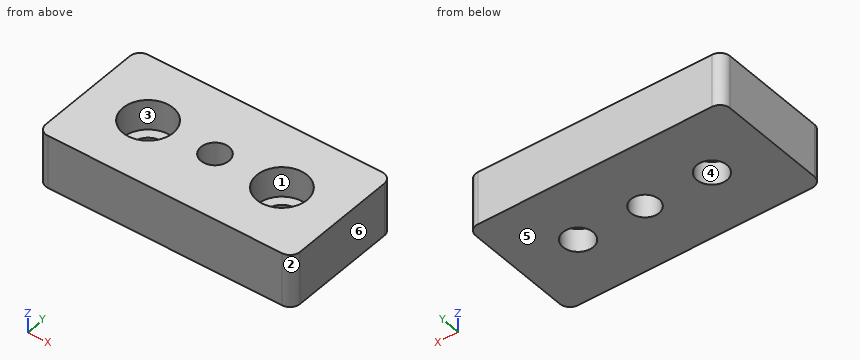
Autodesk Inventor part; units mm, degrees
ref_plane "YZ Plane" through (0, 0, 0) normal (1, 0, 0) x (0, 1, 0)
ref_plane "XZ Plane" through (0, 0, 0) normal (0, 1, 0) x (-1, 0, 0)
ref_plane "XY Plane" through (0, 0, 0) normal (0, 0, 1) x (1, 0, 0)
sketch "Sketch1" plane through (0, 0, 0) normal (0, 0, 1) x (1, 0, 0)
  line L0 (-38, 19) -> (38, 19)
  line L1 (38, 19) -> (38, -19)
  line L2 (38, -19) -> (-38, -19)
  line L3 (-38, -19) -> (-38, 19)
  point P0 (0, 0)
  point P1 (0, 19)
  point P2 (-38, 0)
  dimension "Dim_A" = 76
  dimension "Dim_B" = 38
extrude "Base" add sketch "Sketch1" against normal mid plane 15.9
sketch "Sketch2" plane through (0, 0, 7.95) normal (0, 0, 1) x (1, 0, 0)
  line L0 (0, -26.6) -> (0, 26.6) construction
  line L1 (-53.2, 0) -> (53.2, 0) construction
  point P0 (0, 0)
  point P1 (0, 0)
  point P2 (-20, 0)
  dimension "Dim_D1" = 0
  dimension "Dim_D" = 40
hole "MountHole" at (-20, 0, 7.95) direction (0, 0, -1) diameter 9 end through all counterbore diameter 15 counterbore depth 9
hole "CenterHole" at (0, 0, 7.95) direction (0, 0, -1) diameter 8.376 end through all
pattern_linear "Mount Hole Pattern" count 2 spacing 40 along (1, 0, 0) of "MountHole"
fillet "Fillet1" radius 3 4 edges at (-38, -19, 0) (-38, 19, 0) (38, 19, 0) (38, -19, 0)
properties part number "21-002" material "Steel, High Strength Low Alloy"
Verification items for the finished model (mm, model axes). Face numbers are marked on the shaded views. A direction names the side the tool comes from. Give positions to 0.01 mm unless a question says otherwise; leave off trailing zeros. Order: outer loops, then holes, each group sorted by start corner. A loop starts at its lowest first (then second) coordinate and runs counter-clockwise, first axis right, second up. Notation, with made-up numbers: M 45.25,-36 L 96.25,-36 A10 ccw 96.25,-19 Z; hole C 20,29.25 d8. An arc over 180 degrees is marked long. Use one line per item in the form item = value. Start each with the question number.
Q1. Scan lines: line 1 along X through (y, z) = (0, -3.25); line 2 along X through (y, z) = (0, 4); line 3 along Y through (x, z) = (0, -2.5). Record each from-to range of solid material in increasing order. Write a range as [from, to].
Q2. Section check C-C (z = -4.5). Enter the section's corners in (x, y).
Q3. Section check A-A (x = 0). Enter the section's corners in (y, z), then the cut area to 3 significant figures.
Q4. Mould release check, pull along X, two halves, no side actions. Record for the marked faces 3, 4, 5 and 6: +X half, -X half, draft (parallel to the pull), parting line (faces both ways), or undercut.
Q5. Section check B-B (y = 0). Enter the section's corners in (x, z).
Q6. Access from +Z, -Z, +X, -X, +Y, -Y to the whole of each face (thin tool, end or side, straight path). Record for the marked faces 1 and 2.
Q7. Go/stop test with flat-tipped pins: pin 1 Ø8 at (x, y) = (20, 0) entering from -Z; pin 2 Ø6 at (x, y) = (-21, 1.5) entering from +Z. Record where each tip stops, or that it passes through.
Q8. Section check D-D (x = -20). Enter the section's corners in (y, z), then the cut area to 3 significant figures.
Evaluation:
q1.line_1 = [-38, -24.5], [-15.5, -4.19], [4.19, 15.5], [24.5, 38]
q1.line_2 = [-38, -27.5], [-12.5, -4.19], [4.19, 12.5], [27.5, 38]
q1.line_3 = [-19, -4.19], [4.19, 19]
q2.outline = M -38,-16 A3 ccw -35,-19 L 35,-19 A3 ccw 38,-16 L 38,16 A3 ccw 35,19 L -35,19 A3 ccw -38,16 Z; hole C -20,0 d9; hole C 0,0 d8.38; hole C 20,0 d9
q3.outline = M -19,-7.95 L -4.19,-7.95 L -4.19,7.95 L -19,7.95 Z; M 4.19,-7.95 L 19,-7.95 L 19,7.95 L 4.19,7.95 Z
q3.area = 471 mm2
q4.face_3 = undercut
q4.face_4 = undercut
q4.face_5 = draft
q4.face_6 = +X half
q5.outline = M -38,-7.95 L -24.5,-7.95 L -24.5,-1.05 L -27.5,-1.05 L -27.5,7.95 L -38,7.95 Z; M -15.5,-7.95 L -4.19,-7.95 L -4.19,7.95 L -12.5,7.95 L -12.5,-1.05 L -15.5,-1.05 Z; M 4.19,-7.95 L 15.5,-7.95 L 15.5,-1.05 L 12.5,-1.05 L 12.5,7.95 L 4.19,7.95 Z; M 24.5,-7.95 L 38,-7.95 L 38,7.95 L 27.5,7.95 L 27.5,-1.05 L 24.5,-1.05 Z
q6.face_1 = +Z
q6.face_2 = +Z, -Z, +X, -Y
q7.pin_1 = through
q7.pin_2 = -1.05
q8.outline = M -19,-7.95 L -4.5,-7.95 L -4.5,-1.05 L -7.5,-1.05 L -7.5,7.95 L -19,7.95 Z; M 4.5,-7.95 L 19,-7.95 L 19,7.95 L 7.5,7.95 L 7.5,-1.05 L 4.5,-1.05 Z
q8.area = 407 mm2
